For this review, take the finished solid that the model builds, in its own axes (mm). A direction names the side the tool comes from. Coordinates: 2 decimals unless noted, no trailing zeros. Write each loop counter-clockwise with the first axis right and the second up, starting at its lowest first coordinate (ties: lowest second). Pieces come first, ordered by that corner, then holes. Notation, with made-up numbers: (8, 61.5) -> (38, 61.5) arc R31 cw to (38, 85.5) -> close; hole circle Ø8 at (80.25, 64.5). An arc over 180 degrees is marked (long way). One line per item, written item: value. Start each with the question number.
1) Add section A-A (y = -8.25). State the section outline as (x, z) points.
2) For probe 1 along Y at (x, z) = (-12, 26); probe 2 along Y at (x, z) = (3, 1); probe 3 along Z at (x, y) = (-22, 11), list the stretches that pass through material, from the lowest coordinate up. Write a range as from..to.
3) Machinability: for faces 1 (the flat face through (-6.932, -1.232, -0.033)), 2 (the flat face through (-1.1, -1.23, 6.87)), 3 (the flat face through (0.94, -1.23, -6.92)), 4 (the flat face through (2.836, -1.232, 6.348)), 5 (the flat face through (0, -9, 2.5)), which of the approach directions +Z, -Z, +X, -X, +Y, -Y give a long, thin tool a straight path to every point of the face, cutting with its end or side? Answer none if there is none.
4) For pin 1 Ø1.2 at (x, y) = (-0.5, -8.5) entering from +Z; pin 2 Ø5 at (x, z) = (-7.5, -3.5) entering from +Y; pin 3 Ø10 at (y, z) = (-2, 36.5) entering from +X; pin 4 Ø2 at (y, z) = (-9, 0.5) entering from -X, all flat-tipped, find the tip position at first contact; note any pin that passes through.
5) Mouldability with a two-part tool opening along Y and no side actions: class faces 6 (the flat face through (-7.6, 5, 17.3)), 7 (the flat face through (-5, 12, 13)), 8 (the flat face through (-2.5, -9, 0)) as released by +Y, released by -Y, zero draft, split by the parting line, or undercut.
from build123d import *

# Parameters (mm, degrees)
ESQUISSE1_R             = 2
BOSS_EXTRU_1_DEPTH      = 5
ESQUISSE2_W             = 10
ESQUISSE2_H             = 10
BOSS_EXTRU_2_DEPTH      = 2.5
BOSS_EXTRU_3_DEPTH      = 7
BOSS_EXTRU_4_START      = 5
ESQUISSE5_R             = 2
BOSS_EXTRU_4_DEPTH      = 5
ESQUISSE6_W             = 5
ESQUISSE6_H             = 5
BOSS_EXTRU_5_DEPTH      = 2.5
ESQUISSE7_R             = 7.071067812
ESQUISSE7_R_2           = 5
ENL_V_MAT_EXTRU_1_DEPTH = 2.5
BOSS_EXTRU_6_DEPTH      = 2.5


# Read off the part's stored shape, not the designer's step: Boss.-Extru.3
with BuildPart() as part:
    # Esquisse1 → Boss.-Extru.1 (new body)
    with BuildSketch(Plane(origin=(0, 0, 0), x_dir=(1, 0, 0), z_dir=(0, 1, 0))):
        with Locations(Location((0, 0, 0), (0, 0, 270))):
            Circle(ESQUISSE1_R)
    extrude(amount=BOSS_EXTRU_1_DEPTH)

    # Esquisse2 → Boss.-Extru.2 (add)
    with BuildSketch(Plane.XZ):
        Rectangle(ESQUISSE2_W, ESQUISSE2_H)
    extrude(amount=BOSS_EXTRU_2_DEPTH)

    # Boss.-Extru.3 outline → Boss.-Extru.3 (add)
    with BuildSketch(Plane(origin=(0, 5, 0), x_dir=(1, 0, 0), z_dir=(0, 1, 0))):
        with BuildLine():
            ThreePointArc((1.9752398, -0.313731942), (0.157353741, 1.993800341), (-2, 0))
            add(Edge.make_bspline(
                [(-2, 0), (-7.431064096, -26.884767596), (-31.670728762, -44.785499484)],
                knots=[0, 0, 0, 1, 1, 1], degree=2))
            add(Edge.make_bspline(
                [(-31.670728762, -44.785499484), (-6.018007313, -27.755724693), (1.9752398, -0.313731942)],
                knots=[0.009012394, 0.009012394, 0.009012394, 1.009012394, 1.009012394, 1.009012394], degree=2))
        make_face()
    extrude(amount=BOSS_EXTRU_3_DEPTH)

    # Esquisse5 → Boss.-Extru.4 (add)
    with BuildSketch(Plane.XZ.offset(2.5).offset(BOSS_EXTRU_4_START)):
        with Locations(Location((0, 0, 0), (0, 0, 180))):
            Circle(ESQUISSE5_R)
    extrude(amount=-BOSS_EXTRU_4_DEPTH)

    # Esquisse6 → Boss.-Extru.5 (add)
    with BuildSketch(Plane.XZ.offset(7.5)):
        Rectangle(ESQUISSE6_W, ESQUISSE6_H)
    extrude(amount=BOSS_EXTRU_5_DEPTH)

    # Esquisse7 → Enlèv. mat.-Extru.1 (cut)
    with BuildSketch(Plane(origin=(0, 0, 0), x_dir=(1, 0, 0), z_dir=(0, 1, 0))):
        Circle(ESQUISSE7_R)
        with Locations(Location((0, 0, 0), (0, 0, 270))):
            Circle(ESQUISSE7_R_2, mode=Mode.SUBTRACT)
    extrude(amount=-ENL_V_MAT_EXTRU_1_DEPTH, mode=Mode.SUBTRACT)

    # Esquisse8 → Boss.-Extru.6 (add)
    with BuildSketch(Plane(origin=(0, 0, 0), x_dir=(1, 0, 0), z_dir=(0, 1, 0))):
        with BuildLine():
            Line((0.480722973, 9.091466817), (-0.480722973, 9.091466817))
            Line((-0.480722973, 9.091466817), (-1.384203057, 4.804579263))
            ThreePointArc((-1.384203057, 4.804579263), (0, 5), (1.384203057, 4.804579263))
            Line((1.384203057, 4.804579263), (0.480722973, 9.091466817))
        make_face()
        with BuildLine():
            ThreePointArc((-3.724002251, 3.336436308), (-2.657499069, 4.235292044), (-1.384203057, 4.804579263))
            Line((-1.384203057, 4.804579263), (-4.46192526, 7.922480352))
            Line((-4.46192526, 7.922480352), (-5.270745059, 7.40268343))
            Line((-5.270745059, 7.40268343), (-3.724002251, 3.336436308))
        make_face()
        with BuildLine():
            ThreePointArc((-4.929206832, 0.838403251), (-4.509599896, 2.159515866), (-3.743401614, 3.314655994))
            Line((-3.743401614, 3.314655994), (-7.98794375, 4.266868977))
            Line((-7.98794375, 4.266868977), (-8.38734283, 3.392306983))
            Line((-8.38734283, 3.392306983), (-4.929206832, 0.838403251))
        make_face()
        with BuildLine():
            ThreePointArc((-4.607625844, -1.941593182), (-4.962215179, -0.613531185), (-4.941763812, 0.760901064))
            Line((-4.941763812, 0.760901064), (-8.977846539, -0.714736526))
            Line((-8.977846539, -0.714736526), (-8.841018515, -1.666396338))
            Line((-8.841018515, -1.666396338), (-4.607625844, -1.941593182))
        make_face()
        with BuildLine():
            ThreePointArc((-2.816176348, -4.131482879), (-3.827716111, -3.216922344), (-4.554529885, -2.063069927))
            Line((-4.554529885, -2.063069927), (-7.117346486, -5.440711607))
            Line((-7.117346486, -5.440711607), (-6.487733289, -6.167323972))
            Line((-6.487733289, -6.167323972), (-2.816176348, -4.131482879))
        make_face()
        with BuildLine():
            Line((2.997139213, -8.410592571), (2.670641872, -4.227016914))
            ThreePointArc((2.670641872, -4.227016914), (1.435603167, -4.789472158), (0.094807796, -4.999101067))
            Line((0.094807796, -4.999101067), (2.074638584, -8.681463196))
            Line((2.074638584, -8.681463196), (2.997139213, -8.410592571))
        make_face()
        with BuildLine():
            Line((7.117346486, -5.440711607), (4.554529885, -2.063069927))
            ThreePointArc((4.554529885, -2.063069927), (3.827716111, -3.216922344), (2.816176348, -4.131482879))
            Line((2.816176348, -4.131482879), (6.487733289, -6.167323972))
            Line((6.487733289, -6.167323972), (7.117346486, -5.440711607))
        make_face()
        with BuildLine():
            Line((8.977846539, -0.714736526), (4.941763812, 0.760901064))
            ThreePointArc((4.941763812, 0.760901064), (4.985419694, 0.381563193), (5, 0))
            ThreePointArc((5, 0), (4.900924873, -0.990421825), (4.607625844, -1.941593182))
            Line((4.607625844, -1.941593182), (8.841018515, -1.666396338))
            Line((8.841018515, -1.666396338), (8.977846539, -0.714736526))
        make_face()
        with BuildLine():
            Line((7.98794375, 4.266868977), (3.743401614, 3.314655994))
            ThreePointArc((3.743401614, 3.314655994), (4.509599896, 2.159515866), (4.929206832, 0.838403251))
            Line((4.929206832, 0.838403251), (8.38734283, 3.392306983))
            Line((8.38734283, 3.392306983), (7.98794375, 4.266868977))
        make_face()
        with BuildLine():
            Line((4.46192526, 7.922480352), (1.384203057, 4.804579263))
            ThreePointArc((1.384203057, 4.804579263), (2.657499069, 4.235292044), (3.724002251, 3.336436308))
            Line((3.724002251, 3.336436308), (5.270745059, 7.40268343))
            Line((5.270745059, 7.40268343), (4.46192526, 7.922480352))
        make_face()
        with BuildLine():
            ThreePointArc((-0.094807796, -4.999101067), (-1.435603167, -4.789472158), (-2.670641872, -4.227016914))
            Line((-2.670641872, -4.227016914), (-2.997139213, -8.410592571))
            Line((-2.997139213, -8.410592571), (-2.074638584, -8.681463196))
            Line((-2.074638584, -8.681463196), (-0.094807796, -4.999101067))
        make_face()
    extrude(amount=-BOSS_EXTRU_6_DEPTH)


solid = part.part
Numbers:
1. outline: (-2.5, -2.5) -> (2.5, -2.5) -> (2.5, 2.5) -> (-2.5, 2.5) -> close
2. probe 1: 5..12
2. probe 2: -2.5..0
2. probe 3: 36.56..37.46
3. face 1: -X, +Y, -Y
3. face 2: +Z, -Y
3. face 3: -Z, +Y, -Y
3. face 4: +Y, -Y
3. face 5: +Z, +X, -X, -Y
4. pin 1: z = 2.5
4. pin 2: y = 0
4. pin 3: through
4. pin 4: x = -2.5
5. face 6: undercut
5. face 7: released by +Y
5. face 8: zero draft
